For this review, take the finished solid that the model builds, in its own axes (mm). Give positions to 0.01 mm unless a question says otherwise; leave off trailing zeros. Write each loop counter-clockwise with the first axis right and the second up, starting at its lowest first coordinate (ties: lowest second). Pieces come first, ordered by that corner, then holes. Notation, with made-up numbers: M 30.25,25 L 85.25,25 A22 cw 85.25,36 Z; hole C 35.25,8.25 d11. An arc over 180 degrees is marked long. Use one line per item in the form item = value. Start each with the question number.
Q1. Consider section C-C on z = -2.45. Write out the cut boundary in (x, y).
Q2. Consider section A-A on y = 0.3. Write out the cut boundary in (x, z), and give its area (3 significant figures).
Q3. Consider section B-B on x = -2. Write out the cut boundary in (y, z), and give its area (3 significant figures).
Q4. For probe 1 along X at (y, z) = (0.85, -4.35); probe 2 along X at (y, z) = (1.1, -0.35), list the stretches that pass through material, from the lowest coordinate up. Write a range as [from, to].
```python
from build123d import *

# Parameters (mm, degrees)
BOSS_EXTRUDE1_DEPTH = 2
FILLET1_R           = 2


with BuildPart() as part:
    # Sketch1 → Boss-Extrude1 (new body)
    with BuildSketch(Plane(origin=(0, 0, 0), x_dir=(1, 0, 0), z_dir=(0, 1, 0))):
        with BuildLine():
            Line((0, 5), (-25, 5))
            Line((-25, 5), (-25, 0))
            Line((-25, 0), (-5, 0))
            ThreePointArc((-5, 0), (-3.535533906, 3.535533906), (0, 5))
        make_face()
    extrude(amount=BOSS_EXTRUDE1_DEPTH)

    # Fillet1
    fillet1_edges = [part.edges().sort_by_distance(p)[0] for p in [
        (-25, 1, -5),
    ]]
    fillet(fillet1_edges, radius=FILLET1_R)


solid = part.part
```
Working result:
q1.outline = M -25,0 L -4.36,0 L -4.36,2 L -25,2 Z
q2.outline = M -25,-3 A2 ccw -23,-5 L 0,-5 A5 cw -5,0 L -25,0 Z
q2.area = 105 mm²
q3.outline = M 0,-5 L 2,-5 L 2,-4.58 L 0,-4.58 Z
q3.area = 0.835 mm²
q4.probe_1 = [-24.48, -2.47]
q4.probe_2 = [-25, -4.99]
